The model under review builds one solid part; all positions refer to its coordinate system, in mm. Face numbers are marked on the shaded views. Round coordinates to 2 decimals unless told otherwise and drop trailing zeros. Order: outer loops, then holes, each group sorted by start corner. A loop starts at its lowest first (then second) coordinate and runs counter-clockwise, first axis right, second up. Notation, with made-up numbers: (-19.5, 11) -> (21.5, 11) arc R30 cw to (21.5, 41) -> close; hole circle Ø7 at (0, 16.25). An arc over 180 degrees is marked (long way). Put each result on its own line as item: value. Start each with the question number.
from build123d import *

# Parameters (mm, degrees)
SKETCH1_W            = 80
SKETCH1_H            = 64.62
BOSS_EXTRUDE1_DEPTH  = 10
CUT_EXTRUDE1_DEPTH   = 20
M6_CLEARANCE_HOLE1_D = 7


with BuildPart() as part:
    # Sketch1 → Boss-Extrude1 (new body, symmetric)
    with BuildSketch(Plane.XY):
        Rectangle(SKETCH1_W, SKETCH1_H)
    extrude(amount=BOSS_EXTRUDE1_DEPTH, both=True)

    # Sketch2 → Cut-Extrude1 (cut)
    with BuildSketch(Plane.XY.offset(10)):
        with BuildLine():
            Line((-30.2, 32.31), (30.2, 32.31))
            ThreePointArc((30.2, 32.31), (0, 2.11), (-30.2, 32.31))
        make_face()
    extrude(amount=-CUT_EXTRUDE1_DEPTH, mode=Mode.SUBTRACT)

    # M6 Clearance Hole1 (through all)
    with Locations(Plane(origin=(0, -32.31, 0), x_dir=(-1, 0, 0), z_dir=(0, -1, 0))):
        with Locations((0, 0)):
            Hole(M6_CLEARANCE_HOLE1_D / 2)


solid = part.part
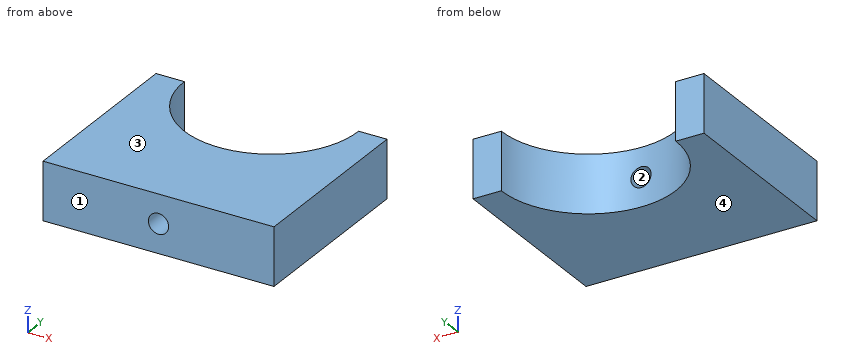
Q1. Take a section at B-B on z = 0. Give the boundary of the cut face in (x, y).
Q2. Wall thickness on probe 1 along Z at (x, y) = (0, -23); probe 2 along X at (y, z) = (23.5, -1); probe 3 along X at (y, z) = (1.5, 2): over which ranges is each line inside the solid? List them lowest first. Write a range as [from, to].
Q3. Take a section at A-A on x = 0. Give the boundary of the cut face in (y, z), and give its area (3 significant figures).
Q4. Take a section at D-D on y = -16.5. Give the boundary of the cut face in (x, z).
Q5. Draft analysis for pull direction Z (two halves, no side actions). For the marked faces 1, 2, 3 and 4, state which applies: +Z half, -Z half, draft (parallel to the pull), parting line (faces both ways), or undercut.
Q6. Clearance check with flat-ended pins moving along their axes: pin 1 Ø9 at (x, z) = (0, 0) entering from -Y; pin 2 Ø10 at (x, z) = (11.5, -2) entering from +Y. State where each tip first meets the part, or that it passes through.
Q7. Take a section at C-C on y = 19. Give the boundary of the cut face in (x, z).
Calculated:
1. outline: (-40, -32.31) -> (-3.5, -32.31) -> (-3.5, 2.31) arc R30.2 cw to (-30.2, 32.31) -> (-40, 32.31) -> close; (3.5, -32.31) -> (40, -32.31) -> (40, 32.31) -> (30.2, 32.31) arc R30.2 cw to (3.5, 2.31) -> close
2. probe 1: z = [-10, -3.5], [3.5, 10]
2. probe 2: x = [-40, -28.89], [28.89, 40]
2. probe 3: x = [-40, -2.87], [2.87, 40]
3. outline: (-32.31, -10) -> (2.11, -10) -> (2.11, -3.5) -> (-32.31, -3.5) -> close; (-32.31, 3.5) -> (2.11, 3.5) -> (2.11, 10) -> (-32.31, 10) -> close
3. area: 447 mm²
4. outline: (-40, -10) -> (40, -10) -> (40, 10) -> (-40, 10) -> close; hole circle Ø7 at (0, 0)
5. face 1: draft
5. face 2: undercut
5. face 3: +Z half
5. face 4: -Z half
6. pin 1: stops at y = -32.31
6. pin 2: stops at y = 7.02
7. outline: (-40, -10) -> (-27.11, -10) -> (-27.11, 10) -> (-40, 10) -> close; (27.11, -10) -> (40, -10) -> (40, 10) -> (27.11, 10) -> close
